```python
from build123d import *

# Parameters (mm, degrees)
SKETCH1_W           = 160
SKETCH1_H           = 20
BOSS_EXTRUDE1_DEPTH = 2
FILLET1_R           = 2
CUT_EXTRUDE1_DEPTH  = 81.647380615
CUT_EXTRUDE2_DEPTH  = 10


with BuildPart() as part:
    # Sketch1 → Boss-Extrude1 (new body)
    with BuildSketch(Plane.XY):
        Rectangle(SKETCH1_W, SKETCH1_H)
    extrude(amount=BOSS_EXTRUDE1_DEPTH)

    # Fillet1
    fillet1_edges = [part.edges().sort_by_distance(p)[0] for p in [
        (80, -10, 1),
        (-80, -10, 1),
        (-80, 10, 1),
        (80, 10, 1),
    ]]
    fillet(fillet1_edges, radius=FILLET1_R)

    # Sketch2 → Cut-Extrude1 (cut, through all)
    with BuildSketch(Plane.XY.offset(2)):
        with BuildLine():
            Line((-70.99, 0), (-70.99, -5))
            ThreePointArc((-70.99, -5), (-72.995, -7.005), (-75, -5))
            Line((-75, -5), (-75, 0))
            ThreePointArc((-75, 0), (-72.995, 2.005), (-70.99, 0))
        make_face()
        with BuildLine():
            Line((70.99, 0), (70.99, -5))
            ThreePointArc((70.99, -5), (72.995, -7.005), (75, -5))
            Line((75, -5), (75, 0))
            ThreePointArc((75, 0), (72.995, 2.005), (70.99, 0))
        make_face()
    extrude(amount=-CUT_EXTRUDE1_DEPTH, mode=Mode.SUBTRACT)

    # Sketch3 → Cut-Extrude2 (cut)
    with BuildSketch(Plane.XY.offset(2)):
        with BuildLine():
            Line((-58.657225294, 5.668547746), (-53.678372606, -4.331452254))
            ThreePointArc((-53.678372606, -4.331452254), (-54.352599567, -6.342774706), (-56.363922019, -5.668547746))
            Line((-56.363922019, -5.668547746), (-61.342774706, 4.331452254))
            ThreePointArc((-61.342774706, 4.331452254), (-60.668547746, 6.342774706), (-58.657225294, 5.668547746))
        make_face()
        with BuildLine():
            Line((-46.101669738, 5.668547746), (-41.12281705, -4.331452254))
            ThreePointArc((-41.12281705, -4.331452254), (-41.797044011, -6.342774706), (-43.808366463, -5.668547746))
            Line((-43.808366463, -5.668547746), (-48.787219151, 4.331452254))
            ThreePointArc((-48.787219151, 4.331452254), (-48.11299219, 6.342774706), (-46.101669738, 5.668547746))
        make_face()
        with BuildLine():
            Line((-33.546114183, 5.668547746), (-28.567261495, -4.331452254))
            ThreePointArc((-28.567261495, -4.331452254), (-29.241488456, -6.342774706), (-31.252810907, -5.668547746))
            Line((-31.252810907, -5.668547746), (-36.231663595, 4.331452254))
            ThreePointArc((-36.231663595, 4.331452254), (-35.557436634, 6.342774706), (-33.546114183, 5.668547746))
        make_face()
        with BuildLine():
            Line((-20.990558627, 5.668547746), (-16.011705939, -4.331452254))
            ThreePointArc((-16.011705939, -4.331452254), (-16.6859329, -6.342774706), (-18.697255352, -5.668547746))
            Line((-18.697255352, -5.668547746), (-23.67610804, 4.331452254))
            ThreePointArc((-23.67610804, 4.331452254), (-23.001881079, 6.342774706), (-20.990558627, 5.668547746))
        make_face()
        with BuildLine():
            Line((-8.435003071, 5.668547746), (-3.456150384, -4.331452254))
            ThreePointArc((-3.456150384, -4.331452254), (-4.130377344, -6.342774706), (-6.141699796, -5.668547746))
            Line((-6.141699796, -5.668547746), (-11.120552484, 4.331452254))
            ThreePointArc((-11.120552484, 4.331452254), (-10.446325523, 6.342774706), (-8.435003071, 5.668547746))
        make_face()
        with BuildLine():
            Line((4.120552484, 5.668547746), (9.099405172, -4.331452254))
            ThreePointArc((9.099405172, -4.331452254), (8.425178211, -6.342774706), (6.413855759, -5.668547746))
            Line((6.413855759, -5.668547746), (1.435003071, 4.331452254))
            ThreePointArc((1.435003071, 4.331452254), (2.109230032, 6.342774706), (4.120552484, 5.668547746))
        make_face()
        with BuildLine():
            Line((16.67610804, 5.668547746), (21.654960727, -4.331452254))
            ThreePointArc((21.654960727, -4.331452254), (20.980733767, -6.342774706), (18.969411315, -5.668547746))
            Line((18.969411315, -5.668547746), (13.990558627, 4.331452254))
            ThreePointArc((13.990558627, 4.331452254), (14.664785588, 6.342774706), (16.67610804, 5.668547746))
        make_face()
        with BuildLine():
            Line((29.231663595, 5.668547746), (34.210516283, -4.331452254))
            ThreePointArc((34.210516283, -4.331452254), (33.536289322, -6.342774706), (31.52496687, -5.668547746))
            Line((31.52496687, -5.668547746), (26.546114183, 4.331452254))
            ThreePointArc((26.546114183, 4.331452254), (27.220341143, 6.342774706), (29.231663595, 5.668547746))
        make_face()
        with BuildLine():
            Line((41.787219151, 5.668547746), (46.766071839, -4.331452254))
            ThreePointArc((46.766071839, -4.331452254), (46.091844878, -6.342774706), (44.080522426, -5.668547746))
            Line((44.080522426, -5.668547746), (39.101669738, 4.331452254))
            ThreePointArc((39.101669738, 4.331452254), (39.775896699, 6.342774706), (41.787219151, 5.668547746))
        make_face()
        with BuildLine():
            Line((54.342774706, 5.668547746), (59.321627394, -4.331452254))
            ThreePointArc((59.321627394, -4.331452254), (58.647400433, -6.342774706), (56.636077981, -5.668547746))
            Line((56.636077981, -5.668547746), (51.657225294, 4.331452254))
            ThreePointArc((51.657225294, 4.331452254), (52.331452254, 6.342774706), (54.342774706, 5.668547746))
        make_face()
    extrude(amount=-CUT_EXTRUDE2_DEPTH, mode=Mode.SUBTRACT)


solid = part.part
```
The listing builds one solid part. Answer for the finished solid, in the listing's coordinates (mm). A direction names the side the tool comes from. Round coordinates to 2 decimals unless told otherwise and drop trailing zeros. Loops run counter-clockwise (first coordinate to the right, second up) from the corner with the lowest first, then second, coordinate; pieces in that order, holes last.
1) For faces 1 (the face through (-1, 0, 0)), 2 (the face through (-5.98, 0.74, 1.01)), determine the directions among +Z, -Z, +X, -X, +Y, -Y from which every point of the face is accessible in a straight line to the end or side of a thin tool.
Outcome:
face 1: -Z, +X, -X, +Y, -Y
face 2: +Z, -Z
2) For a pull along Y with two mould halves and no side action, classify faces 3 (the face through (-1, 0, 2)), 4 (the face through (-56.203, 0.739, 1.014)) as released by +Y, released by -Y, zero draft, split by the parting line, or undercut.
Outcome:
face 3: zero draft
face 4: undercut
3) A cutting plane is placed at A-A on x = -60. Determine the outline of the cut face in (y, z), plus the area to 3 significant figures.
Outcome:
outline: (-10, 0) - (1.63, 0) - (1.63, 2) - (-10, 2) - close; (6.5, 0) - (10, 0) - (10, 2) - (6.5, 2) - close
area: 30.3 mm2
4) Consider line 1 (Y direction, x = 73, z = 1.1) (3 decimals); line 2 (Y direction, x = 56, z = 1.75); line 3 (X direction, y = -9, z = 0.6). Determine where each line is inside the solid, lowest interval first.
Outcome:
line 1: y = -10 to -7.005, 2.005 to 10
line 2: y = -10 to -4.39, 2.34 to 10
line 3: x = -79.73 to 79.73
5) A cutting plane is placed at B-B on z = 1.3. Give the number of separate pieces and of enclosed holes in the cut face, plus the area to 3 significant figures.
Outcome:
separate pieces: 1
enclosed holes: 12
area: 2,730 mm2
